from build123d import *

# Parameters (mm, degrees)
SKETCH1_W          = 7.5
SKETCH1_H          = 2
SKETCH2_R          = 1.125
CUT_EXTRUDE1_DEPTH = 11.793516572
CHAMFER2_SIZE      = 0.1
CHAMFER3_SIZE      = 0.125


with BuildPart() as part:
    # Sketch1 → Revolve1 (revolve)
    with BuildSketch(Plane.XY, mode=Mode.PRIVATE) as revolve1_sk:
        with Locations((3.75, 1)):
            Rectangle(SKETCH1_W, SKETCH1_H)
    revolve(revolve1_sk.sketch.rotate(Axis((0, 0, 0), (0, 1, 0)), 90), axis=Axis((0, 0, 0), (0, 1, 0)))

    # Sketch2 → Cut-Extrude1 (cut, through all)
    with BuildSketch(Plane(origin=(0, 0, 0), x_dir=(1, 0, 0), z_dir=(0, 1, 0))):
        with Locations(Location((-1.732050808, -1, 0), (0, 0, 270))):
            Circle(SKETCH2_R)
        with Locations(Location((1.732050808, -1, 0), (0, 0, 270))):
            Circle(SKETCH2_R)
        with Locations(Location((0, 2, 0), (0, 0, 270))):
            Circle(SKETCH2_R)
    extrude(amount=CUT_EXTRUDE1_DEPTH, mode=Mode.SUBTRACT)

    # Chamfer2
    chamfer2_edges = [part.edges().sort_by_distance(p)[0] for p in [
        (0, 2, -3.125),
        (-1.732050808, 2, -0.125),
        (1.732050808, 2, -0.125),
    ]]
    chamfer(chamfer2_edges, length=CHAMFER2_SIZE)

    # Chamfer3
    chamfer3_edges = [part.edges().sort_by_distance(p)[0] for p in [
        (0, 2, 7.5),
    ]]
    chamfer(chamfer3_edges, length=CHAMFER3_SIZE)


solid = part.part
Can you work these out from the model? Positions are in its coordinate system, mm. Give positions to 0.01 mm unless a question says otherwise; leave off trailing zeros. Loops run counter-clockwise (first coordinate to the right, second up) from the corner with the lowest first, then second, coordinate; pieces in that order, holes last. Notation, with made-up numbers: M 1,1.25 L 22,1.25 A24 cw 22,37.25 Z; hole C 42.25,64 d1. An arc over 180 degrees is marked long. One line per item, written item: value.
1) Thinking about a two-plate mould opening in Z: for faces 1 (the face through (0, 2, 0)), 2 (the face through (-6.324, 0.951, -4.032)), 3 (the face through (-2.73, 0.94, 1.52)), 4 (the face through (0.338, 0.937, -0.927)), which applies, +Z half, -Z half, draft (parallel to the pull), parting line (faces both ways), or undercut?
Geometry check:
face 1: draft
face 2: parting line
face 3: undercut
face 4: undercut
2) Please list where these lines run through material, in increasing order: line 1 (X direction, y = 1.5, z = 2); line 2 (X direction, y = 1.25, z = 1); line 3 (Z direction, x = -1, y = 0.85).
Geometry check:
line 1: x = -7.23 to -2.25, -1.22 to 1.22, 2.25 to 7.23
line 2: x = -7.43 to -2.86, -0.61 to 0.61, 2.86 to 7.43
line 3: z = -7.43 to -2.52, -1.48 to 0.15, 1.85 to 7.43
3) I'm going to push flat-ended pins straight in: pin 1 (2 mm diameter, centred on x = -1.73, z = 1, fed in from -Y) (1 decimal); pin 2 (1 mm diameter, centred on y = 1, z = 0.5, fed in from +X). Where does each tip first touch, or does it pass through?
Geometry check:
pin 1: passes through
pin 2: stops at x = 7.5
4) Imagine slicing it at A-A on x = 0. Write out the boundary of the cut face in (y, z) (3 decimals), and give its area (3 significant figures).
Geometry check:
outline: M 0,-7.5 L 1.875,-7.5 L 2,-7.375 L 2,-3.225 L 1.9,-3.125 L 0,-3.125 Z; M 0,-0.875 L 1.9,-0.875 L 2,-0.775 L 2,7.375 L 1.875,7.5 L 0,7.5 Z
area: 25.5 mm²
5) Imagine slicing it at B-B on z = 1.5. Count the separate pieces of the cut face and the enclosed holes in it, and give its area (3 significant figures).
Geometry check:
separate pieces: 3
enclosed holes: 0
area: 21.3 mm²
